Work out the finished part from the listing and answer in its coordinate system (mm). Give positions to 0.01 mm unless a question says otherwise; leave off trailing zeros. Order: outer loops, then holes, each group sorted by start corner. A loop starts at its lowest first (then second) coordinate and runs counter-clockwise, first axis right, second up. Notation, with made-up numbers: (73, 33.5) -> (86, 33.5) arc R23 ccw to (86, 67.5) -> close; hole circle Ø11 at (48, -29). An arc over 180 degrees is marked (long way). Answer as CSV lines item,"result". Start each with the question number.
1. A flat-ended cylindrical pin translates along its axis: pin 1 (2.5 mm diameter, centred on x = 2, y = 5, fed in from -Z). Find the tip coordinate at first contact, or state that the pin passes through.
2. A cutting plane is placed at A-A (y = 0). Give the vertices of the cut face in (x, z) (3 decimals), then the cut area to 3 significant figures.
3. A cutting plane is placed at C-C (x = 4.5). Give the vertices of the cut face in (y, z) (3 decimals), then the cut area to 3 significant figures.
4. Find the intervals of material crossed by L1, parallel to Z at x = 5.75, y = 3; L2, parallel to X at y = -1, z = 7.5, in increasing order.
5. A cutting plane is placed at B-B (x = 6.35). Give the vertices of the cut face in (y, z) (3 decimals), then the cut area to 3 significant figures.
from build123d import *

# Parameters (mm, degrees)
SKETCH_W     = 9.14
SKETCH_H     = 9.14
PAD_DEPTH    = 7.87
FILLET_R     = 0.7
SKETCH001_R  = 0.35
PAD001_DEPTH = 3.5


with BuildPart() as fillet_body:
    # Sketch → Pad (new body)
    with BuildSketch(Plane.XY.offset(0.1)):
        with Locations((3.175, 3.175)):
            Rectangle(SKETCH_W, SKETCH_H)
    extrude(amount=PAD_DEPTH)

    # Fillet
    fillet_edges = [fillet_body.edges().sort_by_distance(p)[0] for p in [
        (7.745, -1.395, 4.035),
        (7.745, 7.745, 4.035),
        (-1.395, -1.395, 4.035),
        (-1.395, 7.745, 4.035),
    ]]
    fillet(fillet_edges, radius=FILLET_R)


with BuildPart() as obj1:
    # Sketch001 → Pad001 (new body)
    with BuildSketch(Plane.XY.offset(0.5)):
        Circle(SKETCH001_R)
        with Locations((6.35, 6.35)):
            Circle(SKETCH001_R)
    extrude(amount=-PAD001_DEPTH)

    # obj1: union Fillet body
    add(fillet_body.part)


solid = obj1.part
Answer sheet:
1,pin 1,"stops at z = 0.1"
2,outline,"(-1.395, 0.1) -> (-0.35, 0.1) -> (-0.35, -3) -> (0.35, -3) -> (0.35, 0.1) -> (7.745, 0.1) -> (7.745, 7.97) -> (-1.395, 7.97) -> close"
2,area,"74.1 mm^2"
3,outline,"(-1.395, 0.1) -> (7.745, 0.1) -> (7.745, 7.97) -> (-1.395, 7.97) -> close"
3,area,"71.9 mm^2"
4,L1,"z = 0.1 to 7.97"
4,L2,"x = -1.33 to 7.68"
5,outline,"(-1.395, 0.1) -> (6, 0.1) -> (6, -3) -> (6.7, -3) -> (6.7, 0.1) -> (7.745, 0.1) -> (7.745, 7.97) -> (-1.395, 7.97) -> close"
5,area,"74.1 mm^2"
